Source: CAD feature listing. Evaluate the final solid. Frame: model axes, mm. A direction names the side the tool comes from. Give positions to 0.01 mm unless a question says otherwise; leave off trailing zeros. Loops run counter-clockwise (first coordinate to the right, second up) from the corner with the lowest first, then second, coordinate; pieces in that order, holes last. Notation, with made-up numbers: (-15.75, 39) -> (0.25, 39) arc R15 cw to (0.25, 60) -> close; hole circle Ø3 at (60, 37.5). An arc over 180 degrees is marked (long way). Answer as a JSON object with one key per item and string values. Group by question number.
from build123d import *

# Parameters (mm, degrees)
SKETCH1_W           = 35
SKETCH1_H           = 35
BOSS_EXTRUDE1_DEPTH = 1.1
SKETCH2_W           = 25
SKETCH2_H           = 25
BOSS_EXTRUDE2_DEPTH = 5
SKETCH3_W           = 18
SKETCH3_H           = 18
BOSS_EXTRUDE6_DEPTH = 3.1


with BuildPart() as part:
    # Sketch1 → Boss-Extrude1 (new body)
    with BuildSketch(Plane(origin=(0, 0, 0), x_dir=(1, 0, 0), z_dir=(0, 1, 0))):
        Rectangle(SKETCH1_W, SKETCH1_H)
    extrude(amount=BOSS_EXTRUDE1_DEPTH)

    # Sketch2 → Boss-Extrude2 (add)
    with BuildSketch(Plane(origin=(0, 1.1, 0), x_dir=(1, 0, 0), z_dir=(0, 1, 0))):
        Rectangle(SKETCH2_W, SKETCH2_H)
    extrude(amount=BOSS_EXTRUDE2_DEPTH)

    # Sketch3 → Boss-Extrude6 (add)
    with BuildSketch(Plane(origin=(0, 6.1, 0), x_dir=(1, 0, 0), z_dir=(0, 1, 0))):
        Rectangle(SKETCH3_W, SKETCH3_H)
    extrude(amount=BOSS_EXTRUDE6_DEPTH)


solid = part.part
(1) Section query A-A on x = -4.5. Return the cut outline in (y, z), plus the area to 3 significant figures.
(2) Section query B-B on z = 11. Return the cut outline in (x, y), plus the area to 4 significant figures.
(3) Access query for faces 1 (the face through (0, 8, 9)), 2 (the face through (9, 8, 0)), 3 (the face through (0, 8, -9)), 4 (the face through (-9, 8, 0)). Directions: +Z, -Z, +X, -X, +Y, -Y. A direction counts if a zero-diameter tool reaches every point of the face in a straight line with its end or side. Return the directions, or none.
(4) Material intervals for line 1 (Z direction, x = -8, y = 1.75); line 2 (Z direction, x = 7.5, y = 8.75), sorted ascending. Write a range as from..to.
(5) Section query D-D on z = 7. Return the cut outline in (x, y), plus the area to 3 significant figures.
(6) First-contact query: pin 1 (1 mm diameter, centred on x = -12, y = 8, fed in from +Z); pin 2 (4 mm diameter, centred on x = 4.5, y = 4, fed in from -Z); pin 3 (1 mm diameter, centred on x = 0, z = -5, fed in from -Y); pin 4 (2.5 mm diameter, centred on x = -1.5, y = 8.5, fed in from -Z). Flat tips, straight axial feed; report the tip coordinate or a pass-through.
(7) Section query C-C on y = 4.5. Return the cut outline in (x, z).
Result:
{
 "1": {"outline": "(0, -17.5) -> (1.1, -17.5) -> (1.1, -12.5) -> (6.1, -12.5) -> (6.1, -9) -> (9.2, -9) -> (9.2, 9) -> (6.1, 9) -> (6.1, 12.5) -> (1.1, 12.5) -> (1.1, 17.5) -> (0, 17.5) -> close", "area": "219 mm²"},
 "2": {"outline": "(-17.5, 0) -> (17.5, 0) -> (17.5, 1.1) -> (12.5, 1.1) -> (12.5, 6.1) -> (-12.5, 6.1) -> (-12.5, 1.1) -> (-17.5, 1.1) -> close", "area": "163.5 mm²"},
 "3": {"face 1": "+Z, +X, -X, +Y", "face 2": "+Z, -Z, +X, +Y", "face 3": "-Z, +X, -X, +Y", "face 4": "+Z, -Z, -X, +Y"},
 "4": {"line 1": "-12.5..12.5", "line 2": "-9..9"},
 "5": {"outline": "(-17.5, 0) -> (17.5, 0) -> (17.5, 1.1) -> (12.5, 1.1) -> (12.5, 6.1) -> (9, 6.1) -> (9, 9.2) -> (-9, 9.2) -> (-9, 6.1) -> (-12.5, 6.1) -> (-12.5, 1.1) -> (-17.5, 1.1) -> close", "area": "219 mm²"},
 "6": {"pin 1": "through", "pin 2": "z = -12.5", "pin 3": "y = 0", "pin 4": "z = -9"},
 "7": {"outline": "(-12.5, -12.5) -> (12.5, -12.5) -> (12.5, 12.5) -> (-12.5, 12.5) -> close"}
}
